Autodesk Inventor part; units mm, degrees
ref_plane "YZ Plane" through (0, 0, 0) normal (1, 0, 0) x (0, 1, 0)
ref_plane "XZ Plane" through (0, 0, 0) normal (0, 1, 0) x (-1, 0, 0)
ref_plane "XY Plane" through (0, 0, 0) normal (0, 0, 1) x (1, 0, 0)
sketch "Sketch1" plane through (0, 0, 0) normal (0, 0, 1) x (1, 0, 0)
  line L0 (-20, 40) -> (20, 40)
  line L1 (20, 40) -> (20, -40)
  line L2 (20, -40) -> (-20, -40)
  line L3 (-20, -40) -> (-20, 40)
  line L4 (0, 0) -> (10, 0) construction
  line L5 (0, 0) -> (0, -10) construction
  dimension "d0" = 40
  dimension "d1" = 80
  dimension "d2" = 10
  dimension "d3" = 10
extrude "Extrusion1" add sketch "Sketch1" along normal blind 20
sketch "Sketch2" plane through (0, 0, 20) normal (0, 0, 1) x (1, 0, 0)
  line L0 (0, 0) -> (0, 10) construction
  line L1 (0, 0) -> (10, 0) construction
  line L2 (-11, 11) -> (11, 11)
  line L3 (11, 11) -> (11, -11)
  line L4 (11, -11) -> (-11, -11)
  line L5 (-11, -11) -> (-11, 11)
  dimension "d6" = 10
  dimension "d7" = 10
  dimension "d8" = 22
  dimension "d9" = 22
extrude "Extrusion2" cut sketch "Sketch2" against normal blind 15
chamfer "Chamfer1" distance 15 angle 45 1 edges at (0, -11, 20)
chamfer "Chamfer2" distance 15 angle 45 1 edges at (0, 11, 20)
properties part number "rod_socket"
Geometry: final body of the model. Coordinates: model frame, mm. A direction names the side the tool comes from. Round coordinates to 2 decimals unless told otherwise and drop trailing zeros. Write each loop counter-clockwise with the first axis right and the second up, starting at its lowest first coordinate (ties: lowest second). Pieces come first, ordered by that corner, then holes. Notation, with made-up numbers: M -24,-14.5 L 7,-14.5 A22 ccw 7,13.5 Z; hole C 70.5,18.5 d4. An arc over 180 degrees is marked long. Answer in a Markdown table with one row per item. Add a question column.
(1) Reachability of faces 4 (the face through (0, 40, 10)), 5 (the face through (0, -18, 12)) from +Z, -Z, +X, -X, +Y, -Y: full face, straight path, thin tool, end or side. Return the list, or none.
(2) Cut plane A-A, the plane y = -4. Return the cut outline in (x, z).
(3) Ray query, L1, parallel to X at y = 5.5, z = 17; L2, parallel to Y at x = -8, z = 14; L3, parallel to Y at x = -9.5, z = 8.5. Return the intervals inside material, ascending.
(4) Cut plane D-D, the plane z = 8.75. Return the cut outline in (x, y).
(5) Contact query for a flat-ended pin moving along its axis: pin 1 (11 mm diameter, centred on x = -4, y = 1.5, fed in from +Z). Output: stop coordinate, or through.
(6) Cut plane B-B, the plane z = 14. Return the cut outline in (x, y).
(7) Draft query along X for faces 1 (the face through (-11, 0, 14)), 2 (the face through (-14, 1, 20)), 3 (the face through (-20, -1, 10)). Return one class per face: pulls with the +X half, pulls with the -X half, needs draft (parallel to the pull), parting line crosses it, or undercut.
Established:
| question | item | result |
|---|---|---|
| 1 | face 4 | +Z, -Z, +X, -X, +Y |
| 1 | face 5 | +Z |
| 2 | outline | M -20,0 L 20,0 L 20,20 L 11,20 L 11,5 L -11,5 L -11,20 L -20,20 Z |
| 3 | L1 | -20 to -11, 11 to 20 |
| 3 | L2 | -40 to -20, 20 to 40 |
| 3 | L3 | -40 to -14.5, 14.5 to 40 |
| 4 | outline | M -20,-40 L 20,-40 L 20,40 L -20,40 Z; hole M -11,-14.75 L 11,-14.75 L 11,14.75 L -11,14.75 Z |
| 5 | pin 1 | z = 5 |
| 6 | outline | M -20,-40 L 20,-40 L 20,40 L -20,40 Z; hole M -11,-20 L 11,-20 L 11,20 L -11,20 Z |
| 7 | face 1 | undercut |
| 7 | face 2 | needs draft |
| 7 | face 3 | pulls with the -X half |
